from build123d import *

# Parameters (mm, degrees)
F0_R     = 11.2111638742
F0_R_2   = 11.727131611
F1_DEPTH = 10
F2_W     = 22.4031397956
F2_H     = 5
F3_DEPTH = 150


with BuildPart() as f1:
    # F0 (on Front) → F1 (new body)
    with BuildSketch(Plane.XZ):
        with BuildLine():
            ThreePointArc((255, -22.4031397956), (277.4031397956, 0), (255, 22.4031397956))
            Line((255, 22.4031397956), (-255, 22.4031397956))
            ThreePointArc((-255, 22.4031397956), (-277.4031397956, 0), (-255, -22.4031397956))
            Line((-255, -22.4031397956), (255, -22.4031397956))
        make_face()
        with Locations((-255, 0)):
            Circle(F0_R, mode=Mode.SUBTRACT)
        with Locations((255, 0)):
            Circle(F0_R_2, mode=Mode.SUBTRACT)
    extrude(amount=F1_DEPTH)

    # F2 (on face) → F3 (cut)
    with BuildSketch(Plane.XY.offset(22.4031397956)):
        Polygon((-255, 0), (22.4446713773, 0), (22.1150012921, 10.8309555799), (-277.4031397956, 10.8309555799), (-277.4031397956, 0), align=None)
        Polygon((-255, -5), (22.5968602044, -5), (22.4446713773, 0), (-255, 0), align=None)
        with Locations((-266.2015698978, -2.5)):
            Rectangle(F2_W, F2_H)
    extrude(amount=-F3_DEPTH, mode=Mode.SUBTRACT)


solid = f1.part
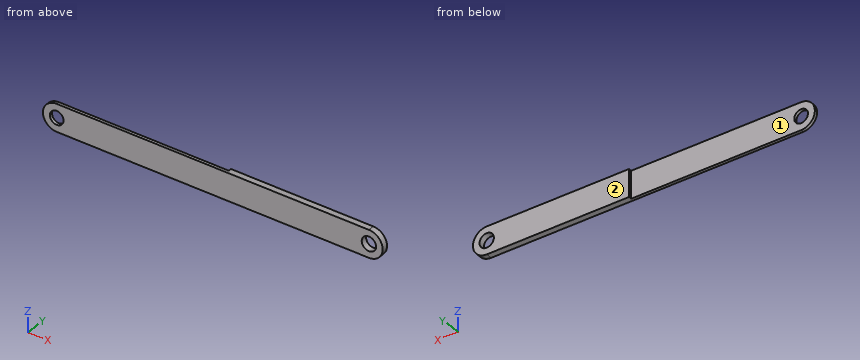
Design review of the part built by this model. Coordinates are the model's own, in mm. Face numbers are marked on the shaded views. A direction names the side the tool comes from. Round coordinates to 2 decimals unless told otherwise and drop trailing zeros. Write each loop counter-clockwise with the first axis right and the second up, starting at its lowest first coordinate (ties: lowest second). Pieces come first, ordered by that corner, then holes. Notation, with made-up numbers: M -3,58 L 26,58 A26 cw 26,86 Z; hole C 52,66 d10. An arc over 180 degrees is marked long. One line per item, written item: value. Start each with the question number.
1. Take a section at B-B on x = -37.5. State the section outline as (y, z) points.
2. Take a section at A-A on z = 0. State the section outline as (x, y) points, then the cut area to 3 significant figures.
3. For the marked faces 1 and 2, list the 3-axis set-ups (+Z, -Z, +X, -X, +Y, -Y) from which the entire face can be reached by the end or side of a thin tool; tool diameter is ignored.
4. To check wall thickness, follow probe 1 along X at (y, z) = (-6.75, -1); probe 2 along X at (y, z) = (-5.5, 6); probe 3 along Z at (x, y) = (-255, -7.3). State the ranges of each line that lie inside material, in increasing order. Write a range as from..to.
5. Clearance check with flat-ended pins moving along their axes: P1, Ø13.5, axis at x = -255, z = 0, coming from the +Y side; P2, Ø22.5, axis at x = -80.5, z = -9, coming from the +Y side; P3, Ø10, axis at x = 200, z = -2.5, coming from the +Y side; P4, Ø5, axis at y = -4.5, z = -5, coming from the +X side. State where each tip first meets the part, or that it passes through.
Computed:
1. outline: M -10,-22.4 L -5,-22.4 L -5,22.4 L -10,22.4 Z
2. outline: M -277.4,-10 L -266.21,-10 L -266.21,-5 L -277.4,-5 Z; M -243.79,-10 L 243.27,-10 L 243.27,0 L 22.44,0 L 22.6,-5 L -243.79,-5 Z; M 266.73,-10 L 277.4,-10 L 277.4,0 L 266.73,0 Z
2. area: 3,700 mm²
3. face 1: +Z, -Z, -X, +Y
3. face 2: +Z, -Z, +X, -X, +Y
4. probe 1: x = -277.38..-266.17, -243.83..243.32, 266.68..277.38
4. probe 2: x = -276.58..-264.47, -245.53..244.92, 265.08..276.58
4. probe 3: z = -22.4..-11.21, 11.21..22.4
5. P1: passes through
5. P2: stops at y = -5
5. P3: stops at y = 0
5. P4: stops at x = 277.26
